```python
from build123d import *

# Parameters (mm, degrees)
BOSS_EXTRUDE1_DEPTH = 34.8615
SKETCH2_R           = 6.35
SKETCH2_R_2         = 5
SKETCH2_W           = 138.882076439
SKETCH2_H           = 152.274276667
CUT_EXTRUDE1_DEPTH  = 318.646799811
SKETCH3_W           = 293.18888876
SKETCH3_H           = 137.971241769
CUT_EXTRUDE2_DEPTH  = 242.109386719


with BuildPart() as part:
    # Sketch1 → Boss-Extrude1 (new body)
    with BuildSketch(Plane.XY):
        with BuildLine():
            add(Edge.make_bspline(
                [(0.000560351, 0.000130087), (0.810633127, 7.359196055), (8.649092025, 17.856605174), (26.286719818, 29.975176328), (52.111128271, 42.069215275), (89.597618475, 49.290763054), (131.400792109, 47.884831915), (173.256699242, 40.041104278), (217.961060472, 29.612974894), (256.952064401, 19.528920948), (290.35983767, 8.71099439), (301.273197721, 4.382828139), (314.816918223, -0.516206742), (309.846313895, 0.000130087)],
                knots=[0, 0, 0, 0, 0.060863618, 0.113688265, 0.188608742, 0.312908923, 0.448482434, 0.557612135, 0.691544113, 0.852438279, 0.92975597, 0.976058229, 1, 1, 1, 1], degree=3))
            add(Edge.make_bspline(
                [(309.846313895, 0.000130087), (303.956832565, 1.47095521), (293.989507544, 2.093987313), (276.26402299, 4.514356704), (260.846344817, 5.427413394), (235.858814759, 7.870306192), (205.101424636, 8.838080282), (157.718638092, 9.030650149), (110.497331172, 6.181495223), (66.506197185, -0.586669107), (36.454672816, -6.098499901), (15.316603331, -6.189065841), (1.230714189, -6.924076091), (0.000560351, 0.000130087)],
                knots=[0, 0, 0, 0, 0.057787081, 0.095274891, 0.171021118, 0.205339302, 0.335319146, 0.464904334, 0.658702312, 0.785511947, 0.893517288, 0.94309214, 1, 1, 1, 1], degree=3))
        make_face()
    extrude(amount=BOSS_EXTRUDE1_DEPTH)

    # Sketch2 → Cut-Extrude1 (cut, through all)
    with BuildSketch(Plane.XY.offset(34.8615)):
        with Locations((20.32, 10.16)):
            Circle(SKETCH2_R)
        with Locations((227.296313895, 19.050130087)):
            Circle(SKETCH2_R_2)
        with Locations((303.087352115, 19.854149729)):
            Rectangle(SKETCH2_W, SKETCH2_H)
    extrude(amount=-CUT_EXTRUDE1_DEPTH, mode=Mode.SUBTRACT)

    # Sketch3 → Cut-Extrude2 (cut, through all)
    with BuildSketch(Plane.XY.offset(34.8615)):
        with Locations((74.351869515, 19.480058122)):
            Rectangle(SKETCH3_W, SKETCH3_H)
    extrude(amount=-CUT_EXTRUDE2_DEPTH, mode=Mode.SUBTRACT)


solid = part.part
```
Input: part model. Units: mm. Frame: model coordinates. Give positions to 0.01 mm unless a question says otherwise; leave off trailing zeros. Order: outer loops, then holes, each group sorted by start corner. A loop starts at its lowest first (then second) coordinate and runs counter-clockwise, first axis right, second up. Notation, with made-up numbers: (28.5, 61.25) -> (63.5, 61.25) arc R30 ccw to (63.5, 98.25) -> close; hole circle Ø2 at (84, 11.25). An arc over 180 degrees is marked (long way). Write each question's results on one line, items separated by ' | '. Start each with the question number.
Item 1: Cut plane A-A on y = 19.5. Return the cut outline in (x, z).
Item 2: Contact query for flat-ended pins moving along their axis: P1, Ø5, axis at x = 224.5, z = 12, coming from the -Y side; P2, Ø5, axis at x = 223.5, z = 18.5, coming from the +Y side. Output: stop coordinate, or through.
Item 3: Mould query, pull axis Y, two halves, no side actions, for faces 1 (the cylindrical face through (232.065, 20.552, 17.675)), 2 (the flat face through (227.4, 13.7, 34.862)). Classes: pulls with the +Y half, pulls with the -Y half, needs draft (parallel to the pull), parting line crosses it, or undercut.
Item 4: Line query: line 1 (X direction, y = 16.5, z = 24); line 2 (X direction, y = 21.25, z = 31); line 3 (Y direction, x = 229.75, z = 6). Output: solid intervals per line, ascending.
Item 5: Cut plane B-B on y = 14.5. Return the cut outline in (x, z).
Established:
1) outline: (220.95, 0) -> (222.32, 0) -> (222.32, 34.86) -> (220.95, 34.86) -> close; (232.28, 0) -> (233.65, 0) -> (233.65, 34.86) -> (232.28, 34.86) -> close
2) P1: y = 8.02 | P2: y = 28.66
3) face 1: undercut | face 2: needs draft
4) line 1: 220.95 to 223, 231.6 to 233.65 | line 2: 220.95 to 222.81, 231.79 to 233.65 | line 3: 7.89 to 14.69, 23.41 to 26.46
5) outline: (220.95, 0) -> (225.22, 0) -> (225.22, 34.86) -> (220.95, 34.86) -> close; (229.37, 0) -> (233.65, 0) -> (233.65, 34.86) -> (229.37, 34.86) -> close
